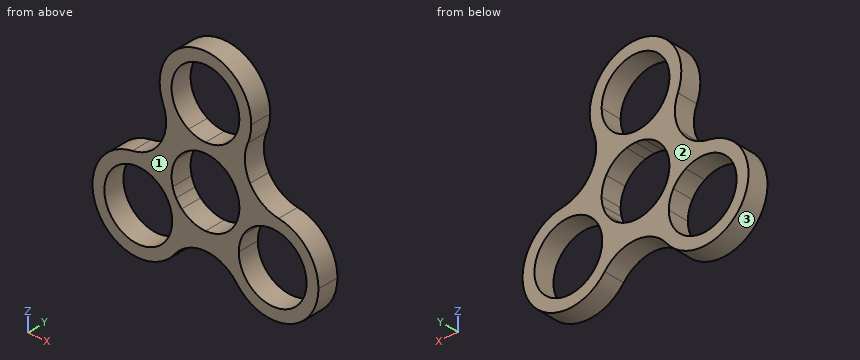
```python
from build123d import *

# Parameters (mm, degrees)
F1_DEPTH = 7


with BuildPart() as f1:
    # F0 (on Front) → F1 (new body)
    with BuildSketch(Plane.XZ):
        with BuildLine():
            Line((-7, 0), (-10.9, 0))
            ThreePointArc((-10.9, 0), (-31.612881982, -5.55), (-16.45, 9.612881982))
            Line((-16.45, 9.612881982), (-14.5, 12.9903810568))
            ThreePointArc((-14.5, 12.9903810568), (-19.0765250841, 14.7123517636), (-23.9637150487, 14.8709052585))
            ThreePointArc((-23.9637150487, 14.8709052585), (-34.9903810568, -7.5), (-10.1032757932, -9.1360797472))
            ThreePointArc((-10.1032757932, -9.1360797472), (-7.7969921654, -4.8243723373), (-7, 0))
        make_face()
        with BuildLine():
            Line((0, 0), (-7, 0))
            ThreePointArc((-7, 0), (-7.7969921654, -4.8243723373), (-10.1032757932, -9.1360797472))
            ThreePointArc((-10.1032757932, -9.1360797472), (-5.6319588622, -5.4687614067), (0, -4.1561539699))
            Line((0, -4.1561539699), (0, 0))
        make_face()
        with BuildLine():
            ThreePointArc((-23.9637150487, 14.8709052585), (-19.0765250841, 14.7123517636), (-14.5, 12.9903810568))
            Line((-14.5, 12.9903810568), (-11, 19.0525588833))
            Line((-11, 19.0525588833), (-14.5993349199, 21.1306358682))
            ThreePointArc((-14.5993349199, 21.1306358682), (-18.5520657365, 16.9095201389), (-23.9637150487, 14.8709052585))
        make_face()
        with BuildLine():
            Line((7, 0), (0, 0))
            Line((0, 0), (0, -4.1561539699))
            ThreePointArc((0, -4.1561539699), (5.6319588622, -5.4687614067), (10.1032757932, -9.1360797472))
            ThreePointArc((10.1032757932, -9.1360797472), (7.7969921654, -4.8243723373), (7, 0))
        make_face()
        with BuildLine():
            Line((-14.5993349199, 21.1306358682), (-11, 19.0525588833))
            Line((-11, 19.0525588833), (-7.5, 25.1147367097))
            ThreePointArc((-7.5, 25.1147367097), (-11.2795329187, 28.2171383402), (-13.8604392555, 32.3702922552))
            ThreePointArc((-13.8604392555, 32.3702922552), (-12.9201068743, 26.6643590343), (-14.5993349199, 21.1306358682))
        make_face()
        with BuildLine():
            Line((10.9, 0), (7, 0))
            ThreePointArc((7, 0), (7.7969921654, -4.8243723373), (10.1032757932, -9.1360797472))
            ThreePointArc((10.1032757932, -9.1360797472), (26.8243723373, -14.2030078346), (37, 0))
            ThreePointArc((37, 0), (33.2795329187, 9.8879794263), (23.9637150487, 14.8709052585))
            ThreePointArc((23.9637150487, 14.8709052585), (19.0765250841, 14.7123517636), (14.5, 12.9903810568))
            Line((14.5, 12.9903810568), (16.45, 9.612881982))
            ThreePointArc((16.45, 9.612881982), (27.55, 9.612881982), (33.1, 0))
            ThreePointArc((33.1, 0), (22, -11.1), (10.9, 0))
        make_face()
        with BuildLine():
            ThreePointArc((-13.8604392555, 32.3702922552), (-11.2795329187, 28.2171383402), (-7.5, 25.1147367097))
            Line((-7.5, 25.1147367097), (-5.55, 28.4922357845))
            ThreePointArc((-5.55, 28.4922357845), (-5.55, 47.7179997485), (11.1, 38.1051177665))
            ThreePointArc((11.1, 38.1051177665), (9.612881982, 32.5551177665), (5.55, 28.4922357845))
            Line((5.55, 28.4922357845), (7.5, 25.1147367097))
            ThreePointArc((7.5, 25.1147367097), (11.2795329187, 28.2171383402), (13.8604392555, 32.3702922552))
            ThreePointArc((13.8604392555, 32.3702922552), (14.7123517636, 35.1816428506), (15, 38.1051177665))
            ThreePointArc((15, 38.1051177665), (-2.9234749159, 52.8174695301), (-13.8604392555, 32.3702922552))
        make_face()
        with BuildLine():
            Line((14.5993349199, 21.1306358682), (11, 19.0525588833))
            Line((11, 19.0525588833), (14.5, 12.9903810568))
            ThreePointArc((14.5, 12.9903810568), (19.0765250841, 14.7123517636), (23.9637150487, 14.8709052585))
            ThreePointArc((23.9637150487, 14.8709052585), (18.5520657365, 16.9095201389), (14.5993349199, 21.1306358682))
        make_face()
        with BuildLine():
            Line((7.5, 25.1147367097), (11, 19.0525588833))
            Line((11, 19.0525588833), (14.5993349199, 21.1306358682))
            ThreePointArc((14.5993349199, 21.1306358682), (12.9201068743, 26.6643590343), (13.8604392555, 32.3702922552))
            ThreePointArc((13.8604392555, 32.3702922552), (11.2795329187, 28.2171383402), (7.5, 25.1147367097))
        make_face()
        with BuildLine():
            Line((11, 19.0525588833), (9.612881982, 18.2517059222))
            ThreePointArc((9.612881982, 18.2517059222), (10.7217766718, 15.5745973228), (11.1, 12.7017059222))
            ThreePointArc((11.1, 12.7017059222), (11.0107964908, 11.2972983465), (10.7446197048, 9.9154633986))
            ThreePointArc((10.7446197048, 9.9154633986), (12.497113483, 11.6058238761), (14.5, 12.9903810568))
            Line((14.5, 12.9903810568), (11, 19.0525588833))
        make_face()
        with BuildLine():
            Line((9.612881982, 7.1517059222), (12.387118018, 5.55))
            ThreePointArc((12.387118018, 5.55), (14.1511147288, 7.8488852712), (16.45, 9.612881982))
            Line((16.45, 9.612881982), (14.5, 12.9903810568))
            ThreePointArc((14.5, 12.9903810568), (12.497113483, 11.6058238761), (10.7446197048, 9.9154633986))
            ThreePointArc((10.7446197048, 9.9154633986), (10.2721252708, 8.4953485406), (9.612881982, 7.1517059222))
        make_face()
        with BuildLine():
            ThreePointArc((7.7852666589, 4.7897135656), (7.1976184329, 2.426829195), (7, 0))
            Line((7, 0), (10.9, 0))
            ThreePointArc((10.9, 0), (11.2782233282, 2.8728914006), (12.387118018, 5.55))
            Line((12.387118018, 5.55), (9.612881982, 7.1517059222))
            ThreePointArc((9.612881982, 7.1517059222), (8.7788749852, 5.9089631776), (7.7852666589, 4.7897135656))
        make_face()
        with BuildLine():
            ThreePointArc((2.9593530459, 23.3999408023), (6.7927427446, 21.4805809074), (9.612881982, 18.2517059222))
            Line((9.612881982, 18.2517059222), (11, 19.0525588833))
            Line((11, 19.0525588833), (7.5, 25.1147367097))
            ThreePointArc((7.5, 25.1147367097), (5.2994950501, 24.0724646954), (2.9593530459, 23.3999408023))
        make_face()
        with BuildLine():
            ThreePointArc((5.55, 28.4922357845), (2.8728914006, 27.3833410947), (0, 27.0051177665))
            Line((0, 27.0051177665), (0, 23.8017059222))
            ThreePointArc((0, 23.8017059222), (1.4932502856, 23.7008060483), (2.9593530459, 23.3999408023))
            ThreePointArc((2.9593530459, 23.3999408023), (5.2994950501, 24.0724646954), (7.5, 25.1147367097))
            Line((7.5, 25.1147367097), (5.55, 28.4922357845))
        make_face()
        with BuildLine():
            Line((-5.55, 28.4922357845), (-7.5, 25.1147367097))
            ThreePointArc((-7.5, 25.1147367097), (-5.2994950501, 24.0724646954), (-2.9593530459, 23.3999408023))
            ThreePointArc((-2.9593530459, 23.3999408023), (-1.4932502856, 23.7008060483), (0, 23.8017059222))
            Line((0, 23.8017059222), (0, 27.0051177665))
            ThreePointArc((0, 27.0051177665), (-2.8728914006, 27.3833410947), (-5.55, 28.4922357845))
        make_face()
        with BuildLine():
            Line((-7.5, 25.1147367097), (-11, 19.0525588833))
            Line((-11, 19.0525588833), (-9.612881982, 18.2517059222))
            ThreePointArc((-9.612881982, 18.2517059222), (-6.7927427446, 21.4805809074), (-2.9593530459, 23.3999408023))
            ThreePointArc((-2.9593530459, 23.3999408023), (-5.2994950501, 24.0724646954), (-7.5, 25.1147367097))
        make_face()
        with BuildLine():
            Line((-11, 19.0525588833), (-14.5, 12.9903810568))
            ThreePointArc((-14.5, 12.9903810568), (-12.497113483, 11.6058238761), (-10.7446197048, 9.9154633986))
            ThreePointArc((-10.7446197048, 9.9154633986), (-10.9991001261, 14.1949562078), (-9.612881982, 18.2517059222))
            Line((-9.612881982, 18.2517059222), (-11, 19.0525588833))
        make_face()
        with BuildLine():
            Line((-14.5, 12.9903810568), (-16.45, 9.612881982))
            ThreePointArc((-16.45, 9.612881982), (-14.1511147288, 7.8488852712), (-12.387118018, 5.55))
            Line((-12.387118018, 5.55), (-9.612881982, 7.1517059222))
            ThreePointArc((-9.612881982, 7.1517059222), (-10.2721252708, 8.4953485406), (-10.7446197048, 9.9154633986))
            ThreePointArc((-10.7446197048, 9.9154633986), (-12.497113483, 11.6058238761), (-14.5, 12.9903810568))
        make_face()
        with BuildLine():
            ThreePointArc((-12.387118018, 5.55), (-11.2782233282, 2.8728914006), (-10.9, 0))
            Line((-10.9, 0), (-7, 0))
            ThreePointArc((-7, 0), (-7.1976184329, 2.426829195), (-7.7852666589, 4.7897135656))
            ThreePointArc((-7.7852666589, 4.7897135656), (-8.7788749852, 5.9089631776), (-9.612881982, 7.1517059222))
            Line((-9.612881982, 7.1517059222), (-12.387118018, 5.55))
        make_face()
        with BuildLine():
            Line((0, 1.6017059222), (0, 0))
            Line((0, 0), (7, 0))
            ThreePointArc((7, 0), (7.1976184329, 2.426829195), (7.7852666589, 4.7897135656))
            ThreePointArc((7.7852666589, 4.7897135656), (4.2063573815, 2.4295806514), (0, 1.6017059222))
        make_face()
        with BuildLine():
            ThreePointArc((-7.7852666589, 4.7897135656), (-7.1976184329, 2.426829195), (-7, 0))
            Line((-7, 0), (0, 0))
            Line((0, 0), (0, 1.6017059222))
            ThreePointArc((0, 1.6017059222), (-4.2063573815, 2.4295806514), (-7.7852666589, 4.7897135656))
        make_face()
    extrude(amount=F1_DEPTH)


solid = f1.part
```
The listing builds one solid part. Answer for the finished solid, in the listing's coordinates (mm). Face numbers are marked on the shaded views. Give positions to 0.01 mm unless a question says otherwise; leave off trailing zeros. Order: outer loops, then holes, each group sorted by start corner. A loop starts at its lowest first (then second) coordinate and runs counter-clockwise, first axis right, second up.
Item 1: The part is cut by section A-A, the plane x = 17.5. Give the vertices of the cut face in (y, z), and give its area (3 significant figures).
From the geometry:
outline: (-7, -14.31) - (0, -14.31) - (0, -10.15) - (-7, -10.15) - close; (-7, 10.15) - (0, 10.15) - (0, 17.69) - (-7, 17.69) - close
area: 82.0 mm2
Item 2: The part is cut by section D-D, the plane y = -2.25. Give the vertices of the cut face in (x, z), and give its area (3 significant figures).
From the geometry:
outline: (-23.96, 14.87) arc R15 ccw (long way) to (-10.1, -9.14) arc R12.74 cw to (10.1, -9.14) arc R15 ccw (long way) to (23.96, 14.87) arc R12.74 cw to (13.86, 32.37) arc R15 ccw (long way) to (-13.86, 32.37) arc R12.74 cw to start; hole circle Ø22.2 at (-22, 0); hole circle Ø22.2 at (0, 12.7); hole circle Ø22.2 at (0, 38.11); hole circle Ø22.2 at (22, 0)
area: 1,280 mm2
Item 3: Given pin 1 Ø8 at (x, z) = (-7.5, 34) entering from -Y; pin 2 Ø1.5 at (x, y) = (-27.5, -1) entering from -Z; pin 3 Ø3 at (y, z) = (-3.5, -2.5) entering from +X, each flat-ended and moving along its own axis, determine where each tip first touches the part or whether it passes through.
From the geometry:
pin 1: stops at y = -7
pin 2: stops at z = -14.23
pin 3: stops at x = 36.97
Item 4: The part is cut by section C-C, the plane x = -6.5. Give the vertices of the cut face in (y, z), and give its area (3 significant figures).
From the geometry:
outline: (-7, -5.94) - (0, -5.94) - (0, 3.7) - (-7, 3.7) - close; (-7, 21.7) - (0, 21.7) - (0, 29.11) - (-7, 29.11) - close; (-7, 47.1) - (0, 47.1) - (0, 51.62) - (-7, 51.62) - close
area: 151 mm2
Item 5: Find the intervals of material crossed by probe 1 along X at (y, z) = (-3.5, 0); probe 2 along Z at (x, y) = (6.5, -2.5); probe 3 along X at (y, z) = (-4.5, -1.5), in increasing order.
From the geometry:
probe 1: x = -37 to -33.1, -10.9 to 10.9, 33.1 to 37
probe 2: z = -5.94 to 3.7, 21.7 to 29.11, 47.1 to 51.62
probe 3: x = -36.92 to -33, -11 to 11, 33 to 36.92
Item 6: The part is cut by section B-B, the plane z = 37. Give the vertices of the cut face in (x, y), and give its area (3 significant figures).
From the geometry:
outline: (-14.96, -7) - (-11.04, -7) - (-11.04, 0) - (-14.96, 0) - close; (11.04, -7) - (14.96, -7) - (14.96, 0) - (11.04, 0) - close
area: 54.8 mm2
Item 7: For a pull along Y with two mould halves and no side action, classify the marked faces 1, 2 and 3 as pulls with the +Y half, pulls with the -Y half, needs draft (parallel to the pull), parting line crosses it, or undercut.
From the geometry:
face 1: pulls with the -Y half
face 2: pulls with the +Y half
face 3: needs draft
